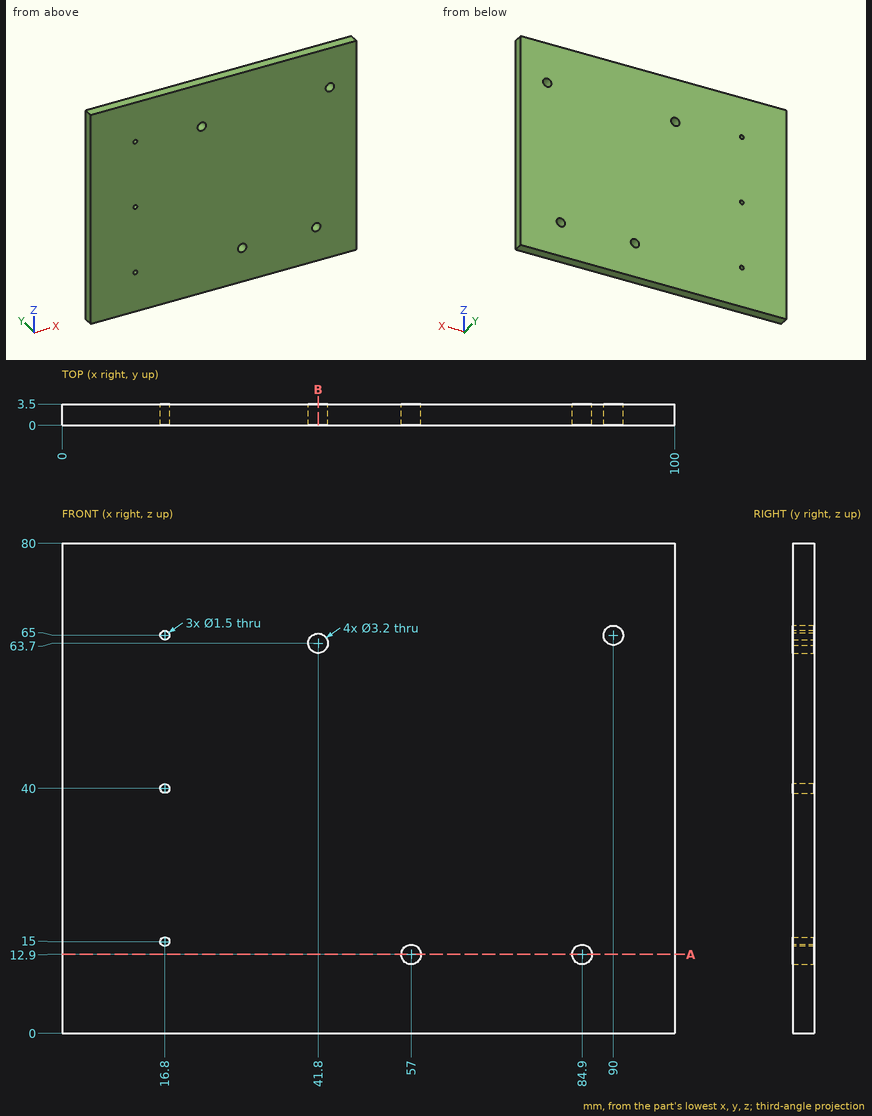
Geometry check sheet. Reference: drawing and pictorial views, mm from the part's lowest x, y, z. Coordinates: 2 decimals unless noted, no trailing zeros. Loops run counter-clockwise (first coordinate to the right, second up) from the corner with the lowest first, then second, coordinate; pieces in that order, holes last. Notation, with made-up numbers: (13, 50) -> (60, 50) arc R8 ccw to (60, 60) -> close; hole circle Ø10 at (31.5, -3.75). An arc over 180 degrees is marked (long way). Write item = value, one per line. Start each with the question number.
1. Section check B-B on x = 41.8. Record the cut outline in (y, z).
2. Depth check by flat-ended pin: P1, Ø1.4, axis at x = 16.8, z = 65, coming from the +Y side. Enter the tip coordinate at first touch or a pass-through.
3. Material ranges on line 1 (Z direction, x = 16.8, y = 2.8); line 2 (Z direction, x = 90, y = 2); line 3 (X direction, y = 1.25, z = 12.9), recorded low to high.
4. Section check A-A on z = 12.9. Record the cut outline in (x, y).
Responses:
q1.outline = (0, 0) -> (3.5, 0) -> (3.5, 62.1) -> (0, 62.1) -> close; (0, 65.3) -> (3.5, 65.3) -> (3.5, 80) -> (0, 80) -> close
q2.P1 = through
q3.line_1 = 0 to 14.25, 15.75 to 39.25, 40.75 to 64.25, 65.75 to 80
q3.line_2 = 0 to 63.4, 66.6 to 80
q3.line_3 = 0 to 55.4, 58.6 to 83.3, 86.5 to 100
q4.outline = (0, 0) -> (55.4, 0) -> (55.4, 3.5) -> (0, 3.5) -> close; (58.6, 0) -> (83.3, 0) -> (83.3, 3.5) -> (58.6, 3.5) -> close; (86.5, 0) -> (100, 0) -> (100, 3.5) -> (86.5, 3.5) -> close
